```python
from build123d import *

# Parameters (mm, degrees)
SKETCH_1_R          = 2.5
EXTRUDE_1_DEPTH     = 180
SKETCH_2_R          = 82.250528809
CUT_EXTRUDE_1_DEPTH = 10


with BuildPart() as part:
    # 草图1 → 凸台-拉伸1 (new, symmetric)
    with BuildSketch(Plane(origin=(0, 0, 0), x_dir=(1, 0, 0), z_dir=(0, 1, 0))):
        Polygon((-15, -3.15), (-12.5, -3.15), (-12.5, -5.15), (-7, -5.15), (-7, -3.15), (-4.5, -3.15), (-4.5, 3.15), (-7, 3.15), (-7, 5.15), (-12.5, 5.15), (-12.5, 3.15), (-15, 3.15), (-15, 15), (-3.15, 15), (-3.15, 12.5), (-5.15, 12.5), (-5.15, 7), (-3.15, 7), (-3.15, 4.5), (3.15, 4.5), (3.15, 7), (5.15, 7), (5.15, 12.5), (3.15, 12.5), (3.15, 15), (15, 15), (15, 3.15), (12.5, 3.15), (12.5, 5.15), (7, 5.15), (7, 3.15), (4.5, 3.15), (4.5, -3.15), (7, -3.15), (7, -5.15), (12.5, -5.15), (12.5, -3.15), (15, -3.15), (15, -15), (3.15, -15), (3.15, -12.5), (5.15, -12.5), (5.15, -7), (3.15, -7), (3.15, -4.5), (-3.15, -4.5), (-3.15, -7), (-5.15, -7), (-5.15, -12.5), (-3.15, -12.5), (-3.15, -15), (-15, -15), align=None)
        with Locations(Location((-9.75, -9.75, 0), (0, 0, 90))):
            Circle(SKETCH_1_R, mode=Mode.SUBTRACT)
        with Locations(Location((-9.75, 9.75, 0), (0, 0, 90))):
            Circle(SKETCH_1_R, mode=Mode.SUBTRACT)
        with Locations(Location((9.75, 9.75, 0), (0, 0, 90))):
            Circle(SKETCH_1_R, mode=Mode.SUBTRACT)
        with Locations(Location((9.75, -9.75, 0), (0, 0, 90))):
            Circle(SKETCH_1_R, mode=Mode.SUBTRACT)
    extrude(amount=EXTRUDE_1_DEPTH, both=True)

    # 草图2 → 切除-拉伸1 (cut)
    with BuildSketch(Plane(origin=(0, 180, 0), x_dir=(1, 0, 0), z_dir=(0, 1, 0))):
        Circle(SKETCH_2_R)
    extrude(amount=-CUT_EXTRUDE_1_DEPTH, mode=Mode.SUBTRACT)


solid = part.part
```
Check sheet for the modelled part. Datum: model origin and axes. Units: mm. A direction names the side the tool comes from. Coordinates: 2 decimals unless noted, no trailing zeros. Answer as a JSON object with one key per item and string values.
1. Sectioned sample at A-A on y = -36. Count the separate pieces of the cut face and the enclosed holes in it, and give its area (3 significant figures).
Outcome:
{"separate pieces": "1", "enclosed holes": "4", "area": "469 mm²"}
2. Release check for a two-part mould opening along Z. For faces 5 (the flat face through (10, -3, -5.15)), 6 (the flat face through (-9, -3, 15)), 7 (the flat face through (9, -3, -15)), 8 (the flat face through (15, -3, 9)) record: pulls with the +Z half, pulls with the -Z half, needs draft (parallel to the pull), parting line crosses it, or undercut.
Outcome:
{"face 5": "undercut", "face 6": "pulls with the +Z half", "face 7": "pulls with the -Z half", "face 8": "needs draft"}
3. Access from +Z, -Z, +X, -X, +Y, -Y to the whole of each face (thin tool, end or side, straight path). Record for faces 1 (the flat face through (0, -3, -4.5)), 2 (the flat face through (-5.15, -3, 10)), 3 (the flat face through (0, 170, 0)), 4 (the flat face through (0, -3, 4.5)).
Outcome:
{"face 1": "-Z, +Y, -Y", "face 2": "+Y, -Y", "face 3": "+Z, -Z, +X, -X, +Y", "face 4": "+Z, +Y, -Y"}
4. Scan lines: L1, parallel to Z at x = 9.75, y = 17.5; L2, parallel to X at y = -41.5, z = -9.5; L3, parallel to Z at x = 3.5, y = -118.5. Record each from-to range of solid material in increasing order. Write a range as from..to.
Outcome:
{"L1": "-15..-12.25, -7.25..-5.15, 5.15..7.25, 12.25..15", "L2": "-15..-12.24, -7.26..-5.15, 5.15..7.26, 12.24..15", "L3": "-15..-12.5, -7..7, 12.5..15"}
